Check sheet for the modelled part. Datum: model origin and axes. Units: mm. A direction names the side the tool comes from. Round coordinates to 2 decimals unless told otherwise and drop trailing zeros. Order: outer loops, then holes, each group sorted by start corner. A loop starts at its lowest first (then second) coordinate and runs counter-clockwise, first axis right, second up.
(1) Depth check by flat-ended pin: pin 1 (1 mm diameter, centred on x = 164.5, y = -6.5, fed in from +Z); pin 2 (2 mm diameter, centred on y = 2.5, z = 0.5, fed in from +X); pin 3 (3.5 mm diameter, centred on x = -173.5, y = 3, fed in from -Z). Enter the tip coordinate at first touch or a pass-through.
(2) Thickness scan on probe 1 along X at (y, z) = (13, 1.25); probe 2 along X at (y, z) = (8.5, 8.5); probe 3 along X at (y, z) = (6, 9.5). Record the ranges inside material, lowest first.
(3) Tool access check on faces 4 (the flat face through (212.5, 0, 0)), 5 (the cylindrical face through (125, 13, 0)), 6 (the flat face through (217.5, -4, 4)), 7 (the flat face through (155, 7, 0)). Record the directions out of +Z, -Z, +X, -X, +Y, -Y that give a thin tool (end or side, any length) a straight path to the whole face; none if there is none.
(4) Sectioned sample at A-A, the plane x = -99.5. Enter the section's corners in (y, z).
(5) Mould release check, pull along Z, two halves, no side actions. Record for faces 1 (the cylindrical face through (-40.07, -7.659, -4.727)), 2 (the flat face through (205, 6.5, -6.5)), 3 (the cylindrical face through (-215.04, -4.88, -1.08)): released by +Z, released by -Z, zero draft, split by the parting line, or undercut.
```python
from build123d import *

# Parameters (mm, degrees)
BOSS_EXTRUDE1_DEPTH      = 5
BOSS_EXTRUDE1_DEPTH_BACK = 5
BOSS_EXTRUDE2_DEPTH      = 5
BOSS_EXTRUDE2_DEPTH_BACK = 5
BOSS_EXTRUDE3_DEPTH      = 5
BOSS_EXTRUDE3_DEPTH_BACK = 5
BOSS_EXTRUDE4_DEPTH      = 5
BOSS_EXTRUDE4_DEPTH_BACK = 5
BOSS_EXTRUDE5_DEPTH      = 5
BOSS_EXTRUDE5_DEPTH_BACK = 5
BOSS_EXTRUDE6_DEPTH      = 5
BOSS_EXTRUDE6_DEPTH_BACK = 5
BOSS_EXTRUDE7_DEPTH      = 5
BOSS_EXTRUDE7_DEPTH_BACK = 5
BOSS_EXTRUDE8_DEPTH      = 5
BOSS_EXTRUDE8_DEPTH_BACK = 5
SKETCH12_R               = 5
CUT_EXTRUDE1_DEPTH       = 5


with BuildPart() as part:
    # Sketch2 → Revolve1 (revolve)
    with BuildSketch(Plane(origin=(0, 0, 0), x_dir=(1, 0, 0), z_dir=(0, 1, 0)), mode=Mode.PRIVATE) as revolve1_sk:
        Polygon((-217.5, 0), (217.5, 0), (217.5, 15), (212.5, 15), (212.5, 8.5), (205, 8.5), (205, 15), (200, 15), (200, 6.5), (96.25, 6.5), (96.25, 8.5), (88.75, 8.5), (88.75, 6.5), (-3.75, 6.5), (-3.75, 8.5), (-11.25, 8.5), (-11.25, 6.5), (-103.75, 6.5), (-103.75, 8.5), (-111.25, 8.5), (-111.25, 6.5), (-200, 6.5), (-200, 15), (-205, 15), (-205, 8.5), (-212.5, 8.5), (-212.5, 15), (-217.5, 15), (-217.5, 6.5), align=None)
    revolve(revolve1_sk.sketch.rotate(Axis((-217.5, 0, 0), (1, 0, 0)), 180), axis=Axis((-217.5, 0, 0), (1, 0, 0)))

    # Sketch4 → Boss-Extrude1 (add, two sides: drawn at the far end of the back side and taken through both)
    with BuildSketch(Plane(origin=(-175, 0, 0), x_dir=(0, 0, -1), z_dir=(1, 0, 0)).offset(-BOSS_EXTRUDE1_DEPTH_BACK)):
        with BuildLine():
            Line((-4.5, 7.794228634), (1.5, 11.258330249))
            ThreePointArc((1.5, 11.258330249), (6.5, 11.258330249), (9, 6.92820323))
            Line((9, 6.92820323), (9, 0))
            ThreePointArc((9, 0), (-4.5, -7.794228634), (-4.5, 7.794228634))
        make_face()
    extrude(amount=BOSS_EXTRUDE1_DEPTH + BOSS_EXTRUDE1_DEPTH_BACK)

    # Sketch5 → Boss-Extrude2 (add, two sides: drawn at the far end of the back side and taken through both)
    with BuildSketch(Plane(origin=(-140, 0, 0), x_dir=(0, 0, -1), z_dir=(1, 0, 0)).offset(-BOSS_EXTRUDE2_DEPTH_BACK)):
        with BuildLine():
            Line((-4.5, 7.794228634), (1.5, 11.258330249))
            ThreePointArc((1.5, 11.258330249), (6.5, 11.258330249), (9, 6.92820323))
            Line((9, 6.92820323), (9, 0))
            ThreePointArc((9, 0), (-4.5, -7.794228634), (-4.5, 7.794228634))
        make_face()
    extrude(amount=BOSS_EXTRUDE2_DEPTH + BOSS_EXTRUDE2_DEPTH_BACK)

    # Sketch6 → Boss-Extrude3 (add, two sides: drawn at the far end of the back side and taken through both)
    with BuildSketch(Plane(origin=(-75, 0, 0), x_dir=(0, 0, -1), z_dir=(1, 0, 0)).offset(-BOSS_EXTRUDE3_DEPTH_BACK)):
        with BuildLine():
            Line((-8.94352854, -1.006626672), (-9.968626967, 8.101016998))
            ThreePointArc((-9.968626967, 8.101016998), (-7.5, 12.990381057), (-2.031373033, 12.683592693))
            Line((-2.031373033, 12.683592693), (5.34352854, 7.242009579))
            ThreePointArc((5.34352854, 7.242009579), (4.5, -7.794228634), (-8.94352854, -1.006626672))
        make_face()
    extrude(amount=BOSS_EXTRUDE3_DEPTH + BOSS_EXTRUDE3_DEPTH_BACK)

    # Sketch7 → Boss-Extrude4 (add, two sides: drawn at the far end of the back side and taken through both)
    with BuildSketch(Plane(origin=(-40, 0, 0), x_dir=(0, 0, -1), z_dir=(1, 0, 0)).offset(-BOSS_EXTRUDE4_DEPTH_BACK)):
        with BuildLine():
            Line((-9, 0), (-9, 6.92820323))
            ThreePointArc((-9, 6.92820323), (-6.5, 11.258330249), (-1.5, 11.258330249))
            Line((-1.5, 11.258330249), (4.5, 7.794228634))
            ThreePointArc((4.5, 7.794228634), (4.5, -7.794228634), (-9, 0))
        make_face()
    extrude(amount=BOSS_EXTRUDE4_DEPTH + BOSS_EXTRUDE4_DEPTH_BACK)

    # Sketch8 → Boss-Extrude5 (add, two sides: drawn at the far end of the back side and taken through both)
    with BuildSketch(Plane(origin=(25, 0, 0), x_dir=(0, 0, -1), z_dir=(1, 0, 0)).offset(-BOSS_EXTRUDE5_DEPTH_BACK)):
        with BuildLine():
            Line((4.5, 7.794228634), (10.5, 4.330127019))
            ThreePointArc((10.5, 4.330127019), (13, 0), (10.5, -4.330127019))
            Line((10.5, -4.330127019), (4.5, -7.794228634))
            ThreePointArc((4.5, -7.794228634), (-9, 0), (4.5, 7.794228634))
        make_face()
    extrude(amount=BOSS_EXTRUDE5_DEPTH + BOSS_EXTRUDE5_DEPTH_BACK)

    # Sketch9 → Boss-Extrude6 (add, two sides: drawn at the far end of the back side and taken through both)
    with BuildSketch(Plane(origin=(60, 0, 0), x_dir=(0, 0, -1), z_dir=(1, 0, 0)).offset(-BOSS_EXTRUDE6_DEPTH_BACK)):
        with BuildLine():
            Line((4.5, 7.794228634), (10.5, 4.330127019))
            ThreePointArc((10.5, 4.330127019), (13, 0), (10.5, -4.330127019))
            Line((10.5, -4.330127019), (4.5, -7.794228634))
            ThreePointArc((4.5, -7.794228634), (-9, 0), (4.5, 7.794228634))
        make_face()
    extrude(amount=BOSS_EXTRUDE6_DEPTH + BOSS_EXTRUDE6_DEPTH_BACK)

    # Sketch10 → Boss-Extrude7 (add, two sides: drawn at the far end of the back side and taken through both)
    with BuildSketch(Plane(origin=(125, 0, 0), x_dir=(0, 0, -1), z_dir=(1, 0, 0)).offset(-BOSS_EXTRUDE7_DEPTH_BACK)):
        with BuildLine():
            Line((-7.794228634, 4.5), (-4.330127019, 10.5))
            ThreePointArc((-4.330127019, 10.5), (0, 13), (4.330127019, 10.5))
            Line((4.330127019, 10.5), (7.794228634, 4.5))
            ThreePointArc((7.794228634, 4.5), (0, -9), (-7.794228634, 4.5))
        make_face()
    extrude(amount=BOSS_EXTRUDE7_DEPTH + BOSS_EXTRUDE7_DEPTH_BACK)

    # Sketch11 → Boss-Extrude8 (add, two sides: drawn at the far end of the back side and taken through both)
    with BuildSketch(Plane(origin=(160, 0, 0), x_dir=(0, 0, -1), z_dir=(1, 0, 0)).offset(-BOSS_EXTRUDE8_DEPTH_BACK)):
        with BuildLine():
            Line((-7.794228634, 4.5), (-4.330127019, 10.5))
            ThreePointArc((-4.330127019, 10.5), (0, 13), (4.330127019, 10.5))
            Line((4.330127019, 10.5), (7.794228634, 4.5))
            ThreePointArc((7.794228634, 4.5), (0, -9), (-7.794228634, 4.5))
        make_face()
    extrude(amount=BOSS_EXTRUDE8_DEPTH + BOSS_EXTRUDE8_DEPTH_BACK)

    # Sketch12 → Cut-Extrude1 (cut)
    with BuildSketch(Plane.ZY.offset(217.5)):
        Circle(SKETCH12_R)
    cut_extrude1 = extrude(amount=-CUT_EXTRUDE1_DEPTH, mode=Mode.SUBTRACT)

    # Mirror1: Cut-Extrude1 across plane
    add(cut_extrude1.mirror(Plane(origin=(0, 0, 0), x_dir=(0, 0, 1), z_dir=(1, 0, 0))), mode=Mode.SUBTRACT)


solid = part.part
```
Derived:
1. pin 1: stops at z = 6.71
1. pin 2: stops at x = 212.5
1. pin 3: stops at z = -9
2. probe 1: x = -217.5 to -212.5, -205 to -200, 200 to 205, 212.5 to 217.5
2. probe 2: x = -217.5 to -212.5, -205 to -200, -80 to -70, -45 to -35, 200 to 205, 212.5 to 217.5
2. probe 3: x = -217.5 to -212.5, -205 to -200, -80 to -70, 200 to 205, 212.5 to 217.5
3. face 4: +X
3. face 5: +Y
3. face 6: +Z, -Z, +X, +Y, -Y
3. face 7: none
4. outline: circle Ø13 at (0, 0)
5. face 1: split by the parting line
5. face 2: zero draft
5. face 3: undercut
